Autodesk Inventor part; units mm, degrees
ref_plane "Work Plane1" through (2.25, 0, 0) normal (1, 0, 0) x (0, 1, 0)
ref_plane "XZ Plane" through (0, 0, 0) normal (0, 1, 0) x (-1, 0, 0)
ref_plane "XY Plane" through (0, 0, 0) normal (0, 0, 1) x (1, 0, 0)
sketch "Sketch1" plane through (0, 0, 0) normal (0, 1, 0) x (-1, 0, 0)
  line L0 (3, 3) -> (-3, 3)
  line L1 (-3, 3) -> (-3, -3)
  line L2 (-3, -3) -> (3, -3)
  line L3 (3, -3) -> (3, 3)
  point P0 (0, 0)
  dimension "d0" = 6
  dimension "d1" = 6
  dimension "d2" = 3
  dimension "d3" = 3
extrude "Extrusion1" add sketch "Sketch1" along normal blind 3.6
fillet "Fillet1" radius 0.25 4 edges at (3, 1.8, 3) (3, 1.8, -3) (-3, 1.8, 3) (-3, 1.8, -3)
sketch "Sketch2" plane through (0, 3.6, 0) normal (0, 1, 0) x (1, 0, 0)
  circle A0 centre (0, 0) radius 1.75
  dimension "d7" = 3.5
extrude "Extrusion2" add sketch "Sketch2" along normal blind 1
sketch "Sketch3" plane through (0, 4.6, 0) normal (0, 1, 0) x (1, 0, 0)
  line L0 (0.95, -0.95) -> (-0.95, -0.95)
  line L1 (-0.95, -0.95) -> (-0.95, 0.95)
  line L2 (-0.95, 0.95) -> (0.95, 0.95)
  line L3 (0.95, 0.95) -> (0.95, -0.95)
  point P0 (0, 0)
  dimension "d10" = 1.9
  dimension "d11" = 1.9
  dimension "d12" = 0.95
  dimension "d13" = 0.95
extrude "Extrusion3" add sketch "Sketch3" along normal blind 1.1
sketch "Sketch4" plane through (0, 5.7, 0) normal (0, 1, 0) x (1, 0, 0)
  line L0 (-1.4, -1.4) -> (1.4, -1.4)
  line L1 (1.4, -1.4) -> (1.4, 1.4)
  line L2 (1.4, 1.4) -> (-1.4, 1.4)
  line L3 (-1.4, 1.4) -> (-1.4, -1.4)
  point P0 (0, 0)
  dimension "d16" = 2.8
  dimension "d17" = 2.8
  dimension "d18" = 1.4
  dimension "d19" = 1.4
extrude "Extrusion4" add sketch "Sketch4" along normal blind 1.8
fillet "Fillet2" radius 0.25 4 edges at (1.4, 7.5, 0) (0, 7.5, 1.4) (-1.4, 7.5, 0) (0, 7.5, -1.4)
ref_plane "Work Plane1" through (2.25, 0, 0) normal (1, 0, 0) x (0, 1, 0)
sketch "Sketch5" plane through (2.25, 0, 0) normal (1, 0, 0) x (0, 1, 0)
  line L0 (1.1258, -3.3032) -> (1.1258, -2.4976)
  line L1 (1.1258, -2.4976) -> (0.9258, -2.4976)
  line L2 (0.9258, -2.4976) -> (0.9258, -3.1742)
  line L3 (0.9258, -3.1742) -> (-0.1, -4.2)
  line L4 (-0.1, -4.2) -> (-0.1, -5)
  line L5 (-0.1, -5) -> (0.1, -5)
  line L6 (0.1, -5) -> (0.1, -4.329)
  line L7 (0.1, -4.329) -> (1.1258, -3.3032)
  line L8 (0, 0) -> (-0.9994, 0)
  line L9 (0, 2.75) -> (0, -2.75)
  dimension "d24" = 4.2
  dimension "d25" = 5
  dimension "d26" = 0.1
  dimension "d27" = 0.2
  dimension "d28" = 0.2
  dimension "d29" = 45
  dimension "d30" = 45
extrude "Extrusion5" add sketch "Sketch5" along normal mid plane 0.7
mirror "Mirror1" about plane through (0, 0, 0) normal (1, 0, 0) of "Extrusion5"
mirror "Mirror2" about plane through (0, 0, 0) normal (0, 0, 1) of "Extrusion5", "Mirror1"
properties part number "TL3301SPF160QG_Tactile"
Read the model definition and answer for the solid it produces. Units are mm, in the model's axes. A direction names the side the tool comes from. Round coordinates to 2 decimals unless told otherwise and drop trailing zeros. Write each loop counter-clockwise with the first axis right and the second up, starting at its lowest first coordinate (ties: lowest second). Pieces come first, ordered by that corner, then holes. Notation, with made-up numbers: (-17, -30) - (-5, -30) arc R21 cw to (-5, 1) - close; hole circle Ø10 at (72.25, 10). An arc over 180 degrees is marked (long way). One line per question, with ' | ' between items. Start each with the question number.
1. Section D-D (x = 2.05) is taken. Determine the outline of the cut face in (y, z), and give its area (3 significant figures).
2. For faces 1 (the face through (-2.2, 0.4, 3.7)), 2 (the face through (-1.4, 6, 0)), 3 (the face through (-0.95, 5, 0)), 4 (the face through (0.95, 5, 0)), determine the directions among +Z, -Z, +X, -X, +Y, -Y from which every point of the face is accessible in a straight line to the end or side of a thin tool.
3. Find the intervals of material crossed by probe 1 along Z at (x, y) = (-0.8, 1); probe 2 along Y at (x, z) = (-1.75, 1); probe 3 along Z at (x, y) = (-1.3, 6.25), in increasing order. Write a range as [from, to].
4. Section A-A (x = 0) is taken. Determine the outline of the cut face in (y, z).
5. Section B-B (z = 0) is taken. Determine the outline of the cut face in (x, y).
6. Each of these flat-tipped pins is pushed along its axis until it touches: pin 1 (1.5 mm diameter, centred on y = 5.5, z = -0.5, fed in from +X); pin 2 (1.5 mm diameter, centred on x = -0.5, z = -1.5, fed in from -Y); pin 3 (1.1 mm diameter, centred on x = 1, y = 2.5, fed in from -Z). Where does it stop, or does it pass through?
7. For a pull along Y with two mould halves and no side action, classify faces 5 (the face through (0, 2, -3)), 6 (the face through (0, 0, 0)), 7 (the face through (-2.25, 0.61, 3.82)), 8 (the face through (0, 4.6, 1.1)) as +Y half, -Y half, draft (parallel to the pull), parting line (faces both ways), or undercut.
8. Section C-C (y = 3) is taken. Determine the outline of the cut face in (x, z).
Filled in:
1) outline: (-0.1, -5) - (0.1, -5) - (0.1, -4.33) - (1.13, -3.3) - (1.13, -3) - (3.6, -3) - (3.6, 3) - (1.13, 3) - (1.13, 3.3) - (0.1, 4.33) - (0.1, 5) - (-0.1, 5) - (-0.1, 4.2) - (0.93, 3.17) - (0.93, 3) - (0, 3) - (0, -3) - (0.93, -3) - (0.93, -3.17) - (-0.1, -4.2) - close | area: 22.7 mm²
2) face 1: +X, -X, -Y | face 2: +Z, -Z, -X, +Y | face 3: +Z, -Z, -X | face 4: +Z, -Z, +X
3) probe 1: [-3, 3] | probe 2: [0, 3.6] | probe 3: [-1.4, 1.4]
4) outline: (0, -3) - (3.6, -3) - (3.6, -1.75) - (4.6, -1.75) - (4.6, -0.95) - (5.7, -0.95) - (5.7, -1.4) - (7.25, -1.4) arc R0.25 ccw to (7.5, -1.15) - (7.5, 1.15) arc R0.25 ccw to (7.25, 1.4) - (5.7, 1.4) - (5.7, 0.95) - (4.6, 0.95) - (4.6, 1.75) - (3.6, 1.75) - (3.6, 3) - (0, 3) - close
5) outline: (-3, 0) - (3, 0) - (3, 3.6) - (1.75, 3.6) - (1.75, 4.6) - (0.95, 4.6) - (0.95, 5.7) - (1.4, 5.7) - (1.4, 7.25) arc R0.25 ccw to (1.15, 7.5) - (-1.15, 7.5) arc R0.25 ccw to (-1.4, 7.25) - (-1.4, 5.7) - (-0.95, 5.7) - (-0.95, 4.6) - (-1.75, 4.6) - (-1.75, 3.6) - (-3, 3.6) - close
6) pin 1: x = 1.4 | pin 2: y = 0 | pin 3: z = -3
7) face 5: draft | face 6: -Y half | face 7: +Y half | face 8: undercut
8) outline: (-3, -2.75) arc R0.25 ccw to (-2.75, -3) - (2.75, -3) arc R0.25 ccw to (3, -2.75) - (3, 2.75) arc R0.25 ccw to (2.75, 3) - (-2.75, 3) arc R0.25 ccw to (-3, 2.75) - close
